Read the model definition and answer for the solid it produces. Units are mm, in the model's axes. A direction names the side the tool comes from. Round coordinates to 2 decimals unless told otherwise and drop trailing zeros. Write each loop counter-clockwise with the first axis right and the second up, starting at its lowest first coordinate (ties: lowest second). Pieces come first, ordered by that corner, then holes. Notation, with made-up numbers: (16.5, 46.5) - (51.5, 46.5) arc R22 ccw to (51.5, 62.5) - close; hole circle Ø8 at (35.5, 29.25). An arc over 180 degrees is marked (long way). Use one line per item in the form item = value. Start each with the question number.
1) Consider line 1 along X through (y, z) = (102.25, 4.55); line 2 along Z through (x, y) = (84, -1.7); line 3 along Y through (x, z) = (-62, 6.7). Determine where each line is inside the solid, lowest interval first. Write a range as from..to.
2) Each of these flat-tipped pins is pushed along its axis until it touches: pin 1 (4 mm diameter, centred on x = -84, z = 6.75, fed in from +Y); pin 2 (3 mm diameter, centred on x = -45, y = 68.5, fed in from +Z); pin 3 (1.1 mm diameter, centred on y = 67.5, z = 0.5, fed in from -X); pin 4 (2 mm diameter, centred on x = 84, z = 6.75, fed in from +Y). Where does it stop, or does it pass through?
3) For faces 3 (the face through (1, 54, 0)), 4 (the face through (38.67, 64.01, 1.52)), 5 (the face through (-82.383, -1.479, 47.67)), 6 (the face through (-58.503, 15.904, 5.958)), 7 (the face through (-64, 102, 9)), determine the directions among +Z, -Z, +X, -X, +Y, -Y from which every point of the face is accessible in a straight line to the end or side of a thin tool.
4) The part is cut by section C-C, the plane y = 9.5. Give the vertices of the cut face in (x, z), plus the area to 3 significant figures.
5) The part is cut by section D-D, the plane x = 54. Give the vertices of the cut face in (y, z), plus the area to 3 significant figures.
6) For a pull along X with two mould halves and no side action, classify faces 1 (the face through (85.617, -1.479, 47.67)), 2 (the face through (-1, 0, 30)) as released by +X, released by -X, zero draft, split by the parting line, or undercut.
7) The part is cut by section A-A, the plane x = 11. Give the vertices of the cut face in (y, z).
8) The part is cut by section B-B, the plane x = -38.5. Give the vertices of the cut face in (y, z).
Autodesk Fusion 360 part; units mm, degrees
sketch "Sketch13" plane through (0, 0, 0) normal (0, 0, -1) x (1, 0, 0)
  line L0 (0.9482, -57.3251) -> (45.3598, -81.2391)
  arc A0 (44.4116, -85) -> (45.3598, -81.2391) centre (44.4116, -83) ccw
  line L1 (44.4116, -85) -> (-44.4116, -85)
  arc A1 (-45.3598, -81.2391) -> (-44.4116, -85) centre (-44.4116, -83) ccw
  line L2 (-45.3598, -81.2391) -> (-0.9482, -57.3251)
  arc A2 (0.9482, -57.3251) -> (-0.9482, -57.3251) centre (0, -59.086) ccw
  line L3 (65, -25.163) -> (65, -74.837)
  arc A3 (62.0518, -76.598) -> (65, -74.837) centre (63, -74.837) ccw
  line L4 (62.0518, -76.598) -> (15.9259, -51.7609)
  arc A4 (15.9259, -48.2391) -> (15.9259, -51.7609) centre (16.8741, -50) ccw
  line L5 (15.9259, -48.2391) -> (62.0518, -23.402)
  arc A5 (65, -25.163) -> (62.0518, -23.402) centre (63, -25.163) ccw
  line L6 (-62.0518, -23.402) -> (-15.9259, -48.2391)
  arc A6 (-15.9259, -51.7609) -> (-15.9259, -48.2391) centre (-16.8741, -50) ccw
  line L7 (-15.9259, -51.7609) -> (-62.0518, -76.598)
  arc A7 (-65, -74.837) -> (-62.0518, -76.598) centre (-63, -74.837) ccw
  line L8 (-65, -74.837) -> (-65, -25.163)
  arc A8 (-62.0518, -23.402) -> (-65, -25.163) centre (-63, -25.163) ccw
  line L9 (45.3598, -18.7609) -> (0.9482, -42.6749)
  arc A9 (-0.9482, -42.6749) -> (0.9482, -42.6749) centre (0, -40.914) ccw
  line L10 (-0.9482, -42.6749) -> (-45.3598, -18.7609)
  arc A10 (-44.4116, -15) -> (-45.3598, -18.7609) centre (-44.4116, -17) ccw
  line L11 (-44.4116, -15) -> (44.4116, -15)
  arc A11 (45.3598, -18.7609) -> (44.4116, -15) centre (44.4116, -17) ccw
  line L12 (82.8, 0) -> (87, 0)
  line L13 (87, 0) -> (87, 3)
  line L14 (87, 3) -> (-87, 3)
  line L15 (-87, 3) -> (-87, 0)
  line L16 (-87, 0) -> (-82.8, 0)
  line L17 (-82.8, 0) -> (-82.8, -110)
  line L18 (-82.8, -110) -> (82.8, -110)
  line L19 (82.8, -110) -> (82.8, 0)
  line L20 (65.8, -110) -> (50.8, -110)
  line L21 (50.8, -110) -> (50.8, -60)
  line L22 (50.8, -60) -> (65.8, -60)
  line L23 (65.8, -60) -> (65.8, -110)
  line L24 (-38.8, -110) -> (-53.8, -110)
  line L25 (-53.8, -110) -> (-53.8, -2)
  line L26 (-53.8, -2) -> (-38.8, -2)
  line L27 (-38.8, -2) -> (-38.8, -110)
  dimension "d1" = 15
  dimension "d2" = 15
  dimension "d3" = 17
  dimension "d4" = 50
  dimension "d5" = 108
  dimension "d6" = 29
sketch "Sketch14" plane through (0, 0, 0) normal (0, 0, -1) x (1, 0, 0)
  line L0 (-62.0518, -23.402) -> (-15.9259, -48.2391)
  arc A0 (-15.9259, -51.7609) -> (-15.9259, -48.2391) centre (-16.8741, -50) ccw
  line L1 (-15.9259, -51.7609) -> (-62.0518, -76.598)
  arc A1 (-65, -74.837) -> (-62.0518, -76.598) centre (-63, -74.837) ccw
  line L2 (-65, -74.837) -> (-65, -25.163)
  arc A2 (-62.0518, -23.402) -> (-65, -25.163) centre (-63, -25.163) ccw
  line L3 (-0.9482, -42.6749) -> (-45.3598, -18.7609)
  arc A3 (-44.4116, -15) -> (-45.3598, -18.7609) centre (-44.4116, -17) ccw
  line L4 (-44.4116, -15) -> (44.4116, -15)
  arc A4 (45.3598, -18.7609) -> (44.4116, -15) centre (44.4116, -17) ccw
  line L5 (45.3598, -18.7609) -> (0.9482, -42.6749)
  arc A5 (-0.9482, -42.6749) -> (0.9482, -42.6749) centre (0, -40.914) ccw
  line L6 (-82.8, -110) -> (82.8, -110)
  line L7 (82.8, -110) -> (82.8, 0)
  line L8 (82.8, 0) -> (87, 0)
  line L9 (87, 0) -> (87, 3)
  line L10 (87, 3) -> (-87, 3)
  line L11 (-87, 3) -> (-87, 0)
  line L12 (-87, 0) -> (-82.8, 0)
  line L13 (-82.8, 0) -> (-82.8, -110)
  line L14 (44.4116, -85) -> (-44.4116, -85)
  arc A6 (-45.3598, -81.2391) -> (-44.4116, -85) centre (-44.4116, -83) ccw
  line L15 (-45.3598, -81.2391) -> (-0.9482, -57.3251)
  arc A7 (0.9482, -57.3251) -> (-0.9482, -57.3251) centre (0, -59.086) ccw
  line L16 (0.9482, -57.3251) -> (45.3598, -81.2391)
  arc A8 (44.4116, -85) -> (45.3598, -81.2391) centre (44.4116, -83) ccw
  line L17 (62.0518, -76.598) -> (15.9259, -51.7609)
  arc A9 (15.9259, -48.2391) -> (15.9259, -51.7609) centre (16.8741, -50) ccw
  line L18 (15.9259, -48.2391) -> (62.0518, -23.402)
  arc A10 (65, -25.163) -> (62.0518, -23.402) centre (63, -25.163) ccw
  line L19 (65, -25.163) -> (65, -74.837)
  arc A11 (62.0518, -76.598) -> (65, -74.837) centre (63, -74.837) ccw
  line L20 (65.3, -110) -> (51.3, -110)
  line L21 (51.3, -110) -> (51.3, -61)
  line L22 (51.3, -61) -> (65.3, -61)
  line L23 (65.3, -61) -> (65.3, -110)
  line L24 (-39.3, -110) -> (-53.3, -110)
  line L25 (-53.3, -110) -> (-53.3, -3)
  line L26 (-53.3, -3) -> (-39.3, -3)
  line L27 (-39.3, -3) -> (-39.3, -110)
  dimension "d7" = 107
  dimension "d8" = 49
  dimension "d9" = 14
  dimension "d10" = 14
  dimension "d11" = 29.5
  dimension "d12" = 17.5
sketch "Sketch1" plane through (0, 0, 0) normal (0, 1, 0) x (1, 0, 0)
  line L0 (-75, 0) -> (75, 0) construction
  line L1 (-87, -50) -> (87, -50)
  line L2 (87, -50) -> (87, 0)
  line L3 (87, 0) -> (-87, 0)
  line L4 (-87, 0) -> (-87, -50)
  line L5 (0, -100) -> (0, 100) construction
  circle A0 centre (-84, -47) radius 1.75
  circle A1 centre (-84, -47) radius 3
  circle A2 centre (-84, -6.75) radius 1.75
  circle A3 centre (-84, -6.75) radius 3
  circle A4 centre (84, -47) radius 1.75
  circle A5 centre (84, -47) radius 3
  circle A6 centre (84, -6.75) radius 1.75
  circle A7 centre (84, -6.75) radius 3
  line L6 (-87, -5) -> (87, -5) construction
  dimension "d99_1" = 150
  dimension "d100_1" = 174
  dimension "d101_1" = 50
  dimension "d102_1" = 200
  dimension "d103_1" = 3.5
  dimension "d104_1" = 6
  dimension "d105_1" = 3.5
  dimension "d106_1" = 6
  dimension "d107_1" = 3.5
  dimension "d108_1" = 6
  dimension "d109_1" = 3.5
  dimension "d110_1" = 6
  dimension "d111_1" = 5
extrude "Extrude1" add sketch "Sketch1" against normal blind 3 contours A7 | A3 | L1 L2 L3 L4 A1 A5 | A1 | A5
sketch "Sketch2" plane through (0, 0, 0) normal (0, 1, 0) x (-1, 0, 0)
  circle A0 centre (-84, 6.75) radius 1.75
  circle A1 centre (-84, 47) radius 1.75
  circle A2 centre (84, 6.75) radius 1.75
  circle A3 centre (84, 47) radius 1.75
  line L0 (87, 50) -> (-87, 50)
  line L1 (-87, 50) -> (-87, 0)
  line L2 (-87, 0) -> (87, 0)
  line L3 (87, 0) -> (87, 50)
  line L4 (-87, 3) -> (87, 3)
  line L5 (-82.8, 0) -> (-82.8, 1)
  line L6 (-82.8, 1) -> (-80.8, 3)
  line L7 (-82.8, 1) -> (82.8, 1) construction
  line L8 (82.8, 0) -> (82.8, 1)
  line L9 (82.8, 1) -> (80.8, 3)
  line L10 (0, 70.9993) -> (0, -26.0281) construction
  line L11 (0, 100) -> (0, -100)
  point P0 (0, 1)
  dimension "d114_1" = 3
  dimension "d115_1" = 1
  dimension "d116_1" = 45
  dimension "d118_1" = 1
  dimension "d119_1" = 135
  dimension "d18" = 165.6
extrude "Extrude22" add sketch "Sketch2" along normal blind 8 contours L2 L4 L5 L6 L11 | L2 L4 L8 L9 L11
extrude "Extrude2" add sketch "Sketch2" along normal blind 110 contours L2 L4 L5 L6 L11 | L2 L4 L8 L9 L11
sketch "Sketch3" plane through (0, 0, 3) normal (0, 0, 1) x (-1, 0, 0)
  line L0 (80.8, 0) -> (-80.8, 0)
  line L1 (-80.8, 0) -> (-80.8, -110)
  line L2 (-80.8, -110) -> (80.8, -110)
  line L3 (80.8, -110) -> (80.8, 0)
  line L4 (0, 0) -> (0, -110) construction
  curve L5 construction
  curve L6 construction
  curve L7 construction
  curve L8 construction
  circle A0 centre (62, -15.75) radius 1.45
  circle A1 centre (62, -15.75) radius 3.5
  circle A2 centre (62, -102.25) radius 1.45
  circle A3 centre (62, -102.25) radius 3.5
  circle A4 centre (-62, -15.75) radius 1.45
  circle A5 centre (-62, -15.75) radius 3.5
  circle A6 centre (-62, -102.25) radius 1.45
  circle A7 centre (-62, -102.25) radius 3.5
  line L9 (65, -85) -> (-65, -85)
  line L10 (-65, -85) -> (-65, -15)
  line L11 (-65, -15) -> (65, -15)
  line L12 (65, -15) -> (65, -85)
  line L13 (65, -15) -> (-65, -85) construction
  line L14 (65, -85) -> (-65, -15) construction
  line L15 (65, -78.1855) -> (12.6556, -50)
  line L16 (0, -43.1855) -> (-52.3444, -15)
  line L17 (52.3444, -85) -> (0, -56.8145)
  line L18 (-12.6556, -50) -> (-65, -21.8145)
  line L19 (65, -21.8145) -> (12.6556, -50)
  line L20 (0, -56.8145) -> (-52.3444, -85)
  line L21 (52.3444, -15) -> (0, -43.1855)
  line L22 (-12.6556, -50) -> (-65, -78.1855)
  line L23 (73.5, 0) -> (-73.5, 0) construction
  line L24 (-73.5, 0) -> (-73.5, -95) construction
  line L25 (-73.5, -95) -> (73.5, -95) construction
  line L26 (73.5, -95) -> (73.5, 0) construction
  point P0 (0, -55)
  dimension "d124_1" = 2.9
  dimension "d125_1" = 7
  dimension "d126_1" = 2.9
  dimension "d127_1" = 7
  dimension "d128_1" = 2.9
  dimension "d129_1" = 7
  dimension "d130_1" = 2.9
  dimension "d131_1" = 7
  dimension "d132_1" = 86.5
  dimension "d133_1" = 124
  dimension "d134_1" = 15.75
  dimension "d149_1" = 130
  dimension "d150_1" = 70
  dimension "d154_1" = 6
  dimension "d31" = 147
  dimension "d32" = 95
  dimension "d33" = 6
  dimension "d34" = 15
  dimension "d35" = 6
  dimension "d175" = 86.5
extrude "Extrude6" cut sketch "Sketch3" against normal blind 3 contours L11 L16 L21 | L12 L15 L19 | L9 L17 L20 | L10 L18 L22
extrude "Extrude3" add sketch "Sketch3" along normal blind 6 contours A0 A1 L11 L12 | A0 A1 L11 L12 | A4 A5 L10 L11 | A4 A5 L10 L11 | A3 | A7
fillet "Fillet1" radius 2 12 edges at (-52.3444, 85, 1.5) (12.6556, 50, 1.5) (0, 56.8145, 1.5) (-12.6556, 50, 1.5) (0, 43.1855, 1.5) (52.3444, 85, 1.5) (-65, 21.8145, 1.5) (-65, 78.1855, 1.5) (65, 78.1855, 1.5) (65, 21.8145, 1.5) (52.3444, 15, 1.5) (-52.3444, 15, 1.5)
extrude "Extrude31" [suppressed]
chamfer "Chamfer38" [suppressed]
chamfer "Chamfer39" [suppressed]
chamfer "Chamfer40" [suppressed]
chamfer "Chamfer41" [suppressed]
chamfer "Chamfer42" [suppressed]
extrude "Extrude32" [suppressed]
chamfer "Chamfer43" [suppressed]
Geometry results:
q1.line_1 = -65.5..-63.45, -60.55..-58.5, 58.5..60.55, 63.45..65.5
q1.line_2 = 0..5, 8.5..45.25, 48.75..50
q1.line_3 = -3..0, 12.25..14.3, 17.2..19.25, 98.75..100.8, 103.7..105.75
q2.pin_1 = 0
q2.pin_2 = 3
q2.pin_3 = -82.8
q2.pin_4 = through
q3.face_3 = -Z, +X, -X, +Y, -Y
q3.face_4 = +Z, -Z
q3.face_5 = +Y, -Y
q3.face_6 = +Z
q3.face_7 = +Z, +X, -X, +Y
q4.outline = (-82.8, 0) - (82.8, 0) - (82.8, 1) - (80.8, 3) - (-80.8, 3) - (-82.8, 1) - close
q4.area = 493 mm2
q5.outline = (-3, 0) - (27.74, 0) - (27.74, 3) - (0, 3) - (0, 50) - (-3, 50) - close; (72.26, 0) - (110, 0) - (110, 3) - (72.26, 3) - close
q5.area = 346 mm2
q6.face_1 = undercut
q6.face_2 = zero draft
q7.outline = (-3, 0) - (15, 0) - (15, 3) - (0, 3) - (0, 50) - (-3, 50) - close; (37.26, 0) - (62.74, 0) - (62.74, 3) - (37.26, 3) - close; (85, 0) - (110, 0) - (110, 3) - (85, 3) - close
q8.outline = (-3, 0) - (15, 0) - (15, 3) - (0, 3) - (0, 50) - (-3, 50) - close; (22.45, 0) - (36.08, 0) - (36.08, 3) - (22.45, 3) - close; (63.92, 0) - (77.55, 0) - (77.55, 3) - (63.92, 3) - close; (85, 0) - (110, 0) - (110, 3) - (85, 3) - close
